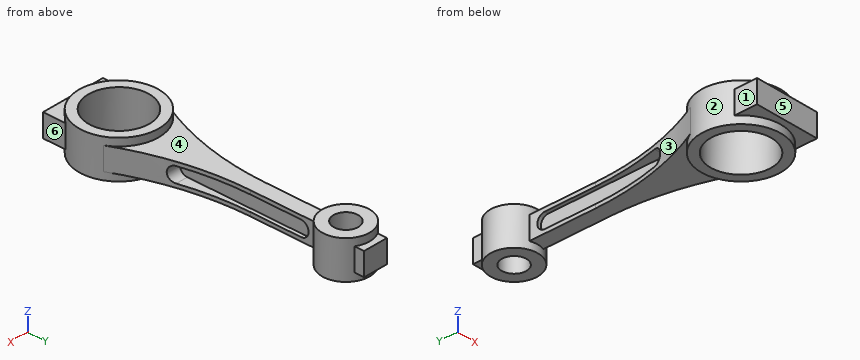
from build123d import *

# Parameters (mm, degrees)
SKETCH1_R             = 21
SKETCH1_R_2           = 16
BOSS_EXTRUDE2_DEPTH   = 10
SKETCH1_R_3           = 12.5
SKETCH1_R_4           = 6.5
BOSS_EXTRUDE2_2_DEPTH = 10
BOSS_EXTRUDE3_DEPTH   = 6
BOSS_EXTRUDE4_DEPTH   = 6
CUT_EXTRUDE1_START    = -6
CUT_EXTRUDE1_DEPTH    = 20
CUT_EXTRUDE6_START    = -2
CUT_EXTRUDE6_DEPTH    = 20


with BuildPart() as part:
    # Sketch1 → Boss-Extrude2 (new body, symmetric)
    with BuildSketch(Plane.XY):
        with Locations((0, -120)):
            Circle(SKETCH1_R)
        with Locations((0, -120)):
            Circle(SKETCH1_R_2, mode=Mode.SUBTRACT)
    extrude(amount=BOSS_EXTRUDE2_DEPTH, both=True)



with BuildPart() as body_2:
    # Sketch1 → Boss-Extrude2 2 (new body, symmetric)
    with BuildSketch(Plane.XY):
        Circle(SKETCH1_R_3)
        Circle(SKETCH1_R_4, mode=Mode.SUBTRACT)
    extrude(amount=BOSS_EXTRUDE2_2_DEPTH, both=True)


with BuildPart() as part_1:
    add(part.part)

    add(body_2.part)  # Boss-Extrude3 merges body 2
    # Sketch1_6 → Boss-Extrude3 (add, symmetric)
    with BuildSketch(Plane.XY):
        with BuildLine():
            ThreePointArc((4, -11.842719282), (0, -12.5), (-4, -11.842719282))
            Line((-4, -11.842719282), (-4, -46.842719282))
            ThreePointArc((-4, -46.842719282), (-7.760864887, -79.642724072), (-18.848249172, -110.740221215))
            ThreePointArc((-18.848249172, -110.740221215), (0, -99), (18.848249172, -110.740221215))
            ThreePointArc((18.848249172, -110.740221215), (7.760864887, -79.642724072), (4, -46.842719282))
            Line((4, -46.842719282), (4, -11.842719282))
        make_face()
        with BuildLine():
            ThreePointArc((17, -132.328828006), (0, -141), (-17, -132.328828006))
            Line((-17, -132.328828006), (-17, -144.328828006))
            Line((-17, -144.328828006), (17, -144.328828006))
            Line((17, -144.328828006), (17, -132.328828006))
        make_face()
    extrude(amount=BOSS_EXTRUDE3_DEPTH, both=True)

    # Sketch2 → Boss-Extrude4 (add, symmetric)
    with BuildSketch(Plane.XY):
        with BuildLine():
            Line((6.5, 15.677078252), (6.5, 10.677078252))
            ThreePointArc((6.5, 10.677078252), (0, 12.5), (-6.5, 10.677078252))
            Line((-6.5, 10.677078252), (-6.5, 15.677078252))
            Line((-6.5, 15.677078252), (6.5, 15.677078252))
        make_face()
    extrude(amount=BOSS_EXTRUDE4_DEPTH, both=True)

    # Sketch3 → Cut-Extrude1 (cut, through all)
    with BuildSketch(Plane(origin=(4, 0, 0), x_dir=(0, 0, -1), z_dir=(1, 0, 0)).offset(CUT_EXTRUDE1_START)):
        with BuildLine():
            Line((-4, -82), (-4, -20))
            ThreePointArc((-4, -20), (0, -16), (4, -20))
            Line((4, -20), (4, -82))
            ThreePointArc((4, -82), (0, -86), (-4, -82))
        make_face()
    extrude(amount=-CUT_EXTRUDE1_DEPTH, mode=Mode.SUBTRACT)

    # Sketch3_5 → Cut-Extrude6 (cut, through all)
    with BuildSketch(Plane(origin=(4, 0, 0), x_dir=(0, 0, -1), z_dir=(1, 0, 0)).offset(CUT_EXTRUDE6_START)):
        with BuildLine():
            Line((-4, -82), (-4, -20))
            ThreePointArc((-4, -20), (0, -16), (4, -20))
            Line((4, -20), (4, -82))
            ThreePointArc((4, -82), (0, -86), (-4, -82))
        make_face()
    extrude(amount=CUT_EXTRUDE6_DEPTH, mode=Mode.SUBTRACT)


solid = part_1.part
Read the model definition and answer for the solid it produces. Units are mm, in the model's axes. Face numbers are marked on the shaded views. A direction names the side the tool comes from. Coordinates: 2 decimals unless noted, no trailing zeros. Loops run counter-clockwise (first coordinate to the right, second up) from the corner with the lowest first, then second, coordinate; pieces in that order, holes last. Notation, with made-up numbers: (63.25, 79.25) -> (120.25, 79.25) arc R24 ccw to (120.25, 116.25) -> close; hole circle Ø9 at (82.5, 72). An arc over 180 degrees is marked (long way). Answer in a Markdown table with one row per item.
Item 1: Each of these flat-tipped pins is pushed along its axis until it touches: P1, Ø1.5, axis at y = 13.5, z = 0.5, coming from the -X side; P2, Ø2.5, axis at y = -61, z = -1, coming from the -X side; P3, Ø5, axis at y = -106.5, z = -4.5, coming from the -X side. Where does it stop, or does it pass through?
Returned:
| item | result |
|---|---|
| P1 | stops at x = -6.5 |
| P2 | stops at x = -2 |
| P3 | stops at x = -18.01 |
Item 2: For a pull along Y with two mould halves and no side action, classify the marked faces 4, 5 and 6 as released by +Y, released by -Y, zero draft, split by the parting line, or undercut.
Returned:
| item | result |
|---|---|
| face 4 | undercut |
| face 5 | released by -Y |
| face 6 | zero draft |
Item 3: A cutting plane is placed at C-C on z = 0. Determine the outline of the cut face in (x, y).
Returned:
| item | result |
|---|---|
| outline | (-18.85, -110.74) arc R21 ccw to (-17, -132.33) -> (-17, -144.33) -> (17, -144.33) -> (17, -132.33) arc R21 ccw to (18.85, -110.74) arc R144.91 cw to (9.39, -86) -> (2, -86) -> (2, -16) -> (4, -16) -> (4, -11.84) arc R12.5 ccw to (6.5, 10.68) -> (6.5, 15.68) -> (-6.5, 15.68) -> (-6.5, 10.68) arc R12.5 ccw to (-4, -11.84) -> (-4, -16) -> (-2, -16) -> (-2, -86) -> (-9.39, -86) arc R144.91 cw to start; hole circle Ø32 at (0, -120); hole circle Ø13 at (0, 0) |
Item 4: A cutting plane is placed at D-D on y = -44. Determine the outline of the cut face in (x, z), plus the area to 3 significant figures.
Returned:
| item | result |
|---|---|
| outline | (-4, -6) -> (4, -6) -> (4, -4) -> (2, -4) -> (2, 4) -> (4, 4) -> (4, 6) -> (-4, 6) -> (-4, 4) -> (-2, 4) -> (-2, -4) -> (-4, -4) -> close |
| area | 64.0 mm^2 |
Item 5: Straight lines are drawn through the part: line 1 along Y through (x, z) = (0, -1); line 2 along Z through (x, y) = (3, -55); line 3 along Y through (x, z) = (-3, -7). For each, find the intervals that lie inside material, in ascending order. Write a range as [from, to].
Returned:
| item | result |
|---|---|
| line 1 | y = [-144.33, -136], [-104, -6.5], [6.5, 15.68] |
| line 2 | z = [-6, -4], [4, 6] |
| line 3 | y = [-140.78, -135.72], [-104.28, -99.22], [-12.13, -5.77], [5.77, 12.13] |
Item 6: A cutting plane is placed at B-B on x = 0. Determine the outline of the cut face in (y, z).
Returned:
| item | result |
|---|---|
| outline | (-144.33, -6) -> (-141, -6) -> (-141, -10) -> (-136, -10) -> (-136, 10) -> (-141, 10) -> (-141, 6) -> (-144.33, 6) -> close; (-104, -10) -> (-99, -10) -> (-99, -6) -> (-12.5, -6) -> (-12.5, -10) -> (-6.5, -10) -> (-6.5, 10) -> (-12.5, 10) -> (-12.5, 6) -> (-99, 6) -> (-99, 10) -> (-104, 10) -> close; (6.5, -10) -> (12.5, -10) -> (12.5, -6) -> (15.68, -6) -> (15.68, 6) -> (12.5, 6) -> (12.5, 10) -> (6.5, 10) -> close |
Item 7: A cutting plane is placed at A-A on y = 0. Determine the outline of the cut face in (x, z).
Returned:
| item | result |
|---|---|
| outline | (-12.5, -10) -> (-6.5, -10) -> (-6.5, 10) -> (-12.5, 10) -> close; (6.5, -10) -> (12.5, -10) -> (12.5, 10) -> (6.5, 10) -> close |
Item 8: For the marked faces 1, 2 and 3, determine the directions among +Z, -Z, +X, -X, +Y, -Y from which every point of the face is accessible in a straight line to the end or side of a thin tool.
Returned:
| item | result |
|---|---|
| face 1 | +Z, -Z, -X, -Y |
| face 2 | none |
| face 3 | +Z, -Z, -X |
